```python
from build123d import *

# Parameters (mm, degrees)
F1_DEPTH = 33.02
F2_W     = 107.3515489697
F2_H     = 51.5172313899
F3_DEPTH = 7.874
F5_R     = 11.0954635734
F4_R     = 12.1126546704
F6_DEPTH = 81.534
F8_DEPTH = 25.4


with BuildPart() as f1:
    # F0 (on Top) → F1 (new body)
    with BuildSketch(Plane.XY):
        with BuildLine():
            ThreePointArc((-47.0562428236, -25.6296646715), (-28.9333331349, -18.1229096887), (-21.4265781521, 0))
            ThreePointArc((-21.4265781521, 0), (-28.9333331349, 18.1229096887), (-47.0562428236, 25.6296646715))
            ThreePointArc((-47.0562428236, 25.6296646715), (-72.6859074951, 0), (-47.0562428236, -25.6296646715))
        make_face()
    extrude(amount=F1_DEPTH)

    # F2 (on Top) → F3 (join)
    with BuildSketch(Plane.XY):
        with Locations((6.0439221561, 0.2878056839)):
            Rectangle(F2_W, F2_H)
    extrude(amount=F3_DEPTH)

    # F5 (on face) + F4 (on face) → F6 (cut)
    with BuildSketch(Plane.XY.offset(33.02)):
        with Locations((-47.0562428236, 0)):
            Circle(F5_R)
    with BuildSketch(Plane.XY.offset(7.874)):
        with Locations((35.8318202198, 0)):
            Circle(F4_R)
    extrude(amount=-F6_DEPTH, mode=Mode.SUBTRACT)

    # F7 (on face) → F8 (cut)
    with BuildSketch(Plane.XY.offset(7.874)):
        with BuildLine():
            ThreePointArc((42.1889192994, 26.0464213789), (53.3155577455, 15.0802409672), (57.3954509182, 0))
            ThreePointArc((57.3954509182, 0), (53.5965706877, -14.5882662321), (43.164924434, -25.470810011))
            Line((43.164924434, -25.470810011), (59.719696641, -25.470810011))
            Line((59.719696641, -25.470810011), (59.719696641, 26.0464213789))
            Line((59.719696641, 26.0464213789), (42.1889192994, 26.0464213789))
        make_face()
    extrude(amount=-F8_DEPTH, mode=Mode.SUBTRACT)


solid = f1.part
```
CAD build for the part. Positions are in the model's coordinates, mm. A direction names the side the tool comes from. Give positions to 0.01 mm unless a question says otherwise; leave off trailing zeros. Loops run counter-clockwise (first coordinate to the right, second up) from the corner with the lowest first, then second, coordinate; pieces in that order, holes last. Notation, with made-up numbers: (39.5, 17.5) -> (82.5, 17.5) arc R16 ccw to (82.5, 39.5) -> close; hole circle Ø2 at (64.5, 56). An arc over 180 degrees is marked (long way). Use a Markdown table: item, result.
1. Flat gauge pins, fed straight in: pin 1 (1.5 mm diameter, centred on x = 12.5, y = -0.5, fed in from +Z); pin 2 (4 mm diameter, centred on x = -40, z = 18, fed in from +Y); pin 3 (4 mm diameter, centred on x = 11, z = 3.5, fed in from -Y). Where does each tip first touch, or does it go through?
Check result:
| item | result |
|---|---|
| pin 1 | stops at z = 7.87 |
| pin 2 | stops at y = 25.13 |
| pin 3 | stops at y = -25.47 |
2. Mould opens along X. For faces 3 (the flat face through (-42, -11, 33.02)), 4 (the cylindrical face through (47.385, 3.638, 3.992)) say: pulls with the +X half, pulls with the -X half, needs draft (parallel to the pull), parting line crosses it, or undercut.
Check result:
| item | result |
|---|---|
| face 3 | needs draft |
| face 4 | undercut |
3. Wall check: L1, parallel to X at y = -7.5, z = 2; L2, parallel to Z at x = 43.5, y = 12; L3, parallel to Y at x = -39, z = 12. Give the ranges that are in metal, low to high. Write a range as [from, to].
Check result:
| item | result |
|---|---|
| L1 | x = [-71.56, -55.23], [-38.88, 26.32], [45.34, 56.44] |
| L2 | z = [0, 7.87] |
| L3 | y = [-24.33, -7.63], [7.63, 24.33] |
4. Slice it at A-A (z = 6.5). List the corners of the cut face in (x, y).
Check result:
| item | result |
|---|---|
| outline | (-47.63, 25.62) arc R25.63 ccw (long way) to (-44.21, -25.47) -> (43.16, -25.47) arc R29.91 ccw to (42.19, 26.05) -> (-47.63, 26.05) -> close; hole circle Ø22.19 at (-47.06, 0); hole circle Ø24.23 at (35.83, 0) |
5. Slice it at C-C (y = 3). List the corners of the cut face in (x, z), plus the area to 3 significant figures.
Check result:
| item | result |
|---|---|
| outline | (-72.51, 0) -> (-57.74, 0) -> (-57.74, 33.02) -> (-72.51, 33.02) -> close; (-36.37, 0) -> (24.1, 0) -> (24.1, 7.87) -> (-21.6, 7.87) -> (-21.6, 33.02) -> (-36.37, 33.02) -> close; (47.57, 0) -> (57.24, 0) -> (57.24, 7.87) -> (47.57, 7.87) -> close |
| area | 1,410 mm^2 |
6. Which spindle directions (+Z, -Z, +X, -X, +Y, -Y) get a long thin tool onto all of the face, cutting with end or side? Do faces 1 (the flat face through (-9, 1, 0)), 2 (the flat face through (-1, -25.471, 4)). Say none if no direction does.
Check result:
| item | result |
|---|---|
| face 1 | -Z, +X, -X, +Y, -Y |
| face 2 | +Z, -Z, +X, -Y |
7. Slice it at D-D (x = -34). List the corners of the cut face in (y, z), plus the area to 3 significant figures.
Check result:
| item | result |
|---|---|
| outline | (-25.47, 0) -> (26.05, 0) -> (26.05, 7.87) -> (22.05, 7.87) -> (22.05, 33.02) -> (-22.05, 33.02) -> (-22.05, 7.87) -> (-25.47, 7.87) -> close |
| area | 1,510 mm^2 |
8. Slice it at B-B (z = 26). List the corners of the cut face in (x, y).
Check result:
| item | result |
|---|---|
| outline | circle Ø51.26 at (-47.06, 0); hole circle Ø22.19 at (-47.06, 0) |
